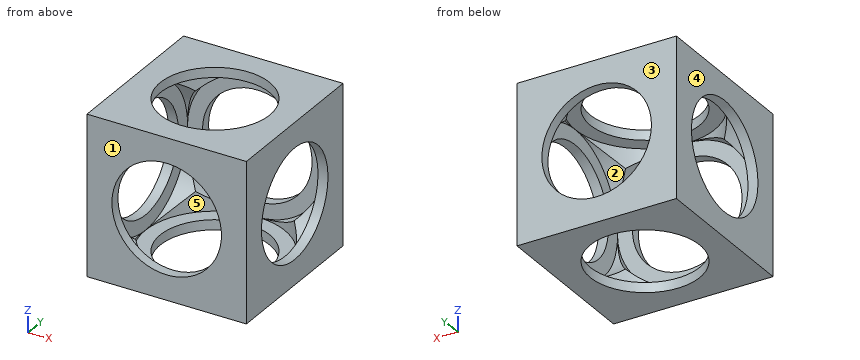
from build123d import *

# Parameters (mm, degrees)
F0_W      = 32
F0_H      = 32
F1_DEPTH  = 16
F2_R      = 11
F3_DEPTH  = 32.001
F4_R      = 11
F5_DEPTH  = 32.001
F6_R      = 11
F7_DEPTH  = 32.001
F8_R      = 14
F9_DEPTH  = 14
F10_R     = 14
F11_DEPTH = 14
F12_R     = 14
F13_DEPTH = 14


with BuildPart() as f1:
    # F0 (on Top) → F1 (new body, symmetric)
    with BuildSketch(Plane.XY):
        Rectangle(F0_W, F0_H)
    extrude(amount=F1_DEPTH, both=True)

    # F2 (on face) → F3 (cut, through all)
    with BuildSketch(Plane(origin=(-16, 0, 0), x_dir=(0, -1, 0), z_dir=(-1, 0, 0))):
        Circle(F2_R)
    extrude(amount=-F3_DEPTH, mode=Mode.SUBTRACT)

    # F4 (on face) → F5 (cut, through all)
    with BuildSketch(Plane.XY.offset(16)):
        Circle(F4_R)
    extrude(amount=-F5_DEPTH, mode=Mode.SUBTRACT)

    # F6 (on face) → F7 (cut, through all)
    with BuildSketch(Plane(origin=(0, 16, 0), x_dir=(-1, 0, 0), z_dir=(0, 1, 0))):
        Circle(F6_R)
    extrude(amount=-F7_DEPTH, mode=Mode.SUBTRACT)

    # F8 (on Top) → F9 (cut, symmetric)
    with BuildSketch(Plane.XY):
        Circle(F8_R)
    extrude(amount=F9_DEPTH, both=True, mode=Mode.SUBTRACT)

    # F10 (on Front) → F11 (cut, symmetric)
    with BuildSketch(Plane.XZ):
        Circle(F10_R)
    extrude(amount=F11_DEPTH, both=True, mode=Mode.SUBTRACT)

    # F12 (on Right) → F13 (cut, symmetric)
    with BuildSketch(Plane.YZ):
        Circle(F12_R)
    extrude(amount=F13_DEPTH, both=True, mode=Mode.SUBTRACT)


solid = f1.part
CAD build for the part. Positions are in the model's coordinates, mm. Face numbers are marked on the shaded views. A direction names the side the tool comes from. Coordinates: 2 decimals unless noted, no trailing zeros. Order: outer loops, then holes, each group sorted by start corner. A loop starts at its lowest first (then second) coordinate and runs counter-clockwise, first axis right, second up. Notation, with made-up numbers: (72.5, 68) -> (120.5, 68) arc R29 ccw to (120.5, 103) -> close; hole circle Ø11 at (9, 80.25). An arc over 180 degrees is marked (long way). Answer in a Markdown table with one row per item.
1) Band-saw the part on C-C (y = -12.5). List the corners of the cut face in (x, z).
Check values:
| item | result |
|---|---|
| outline | (-16, -16) -> (16, -16) -> (16, 16) -> (-16, 16) -> close; hole (-14, -6.3) -> (-12.5, -6.3) arc R14 ccw to (-6.3, -12.5) -> (-6.3, -14) -> (6.3, -14) -> (6.3, -12.5) arc R14 ccw to (12.5, -6.3) -> (14, -6.3) -> (14, 6.3) -> (12.5, 6.3) arc R14 ccw to (6.3, 12.5) -> (6.3, 14) -> (-6.3, 14) -> (-6.3, 12.5) arc R14 ccw to (-12.5, 6.3) -> (-14, 6.3) -> close |
2) Mould opens along Y. For the marked faces 1, 2 and 3 say: pulls with the +Y half, pulls with the -Y half, needs draft (parallel to the pull), parting line crosses it, or undercut.
Check values:
| item | result |
|---|---|
| face 1 | pulls with the -Y half |
| face 2 | undercut |
| face 3 | pulls with the +Y half |
3) Drill centre lines: line 1 (Y direction, x = -11, z = 2); line 2 (Y direction, x = -14.7, z = 0). Where is each one in solid material? Low to high.
Check values:
| item | result |
|---|---|
| line 1 | -16 to -14, 14 to 16 |
| line 2 | -16 to -11, 11 to 16 |
4) Band-saw the part on A-A (z = 2). Give the number of separate pieces and of enclosed holes in the cut face, and give its area (3 significant figures).
Check values:
| item | result |
|---|---|
| separate pieces | 4 |
| enclosed holes | 0 |
| area | 67.0 mm2 |
5) Flat gauge pins, fed straight in: P1, Ø8, axis at y = 7, z = -3.5, coming from the +X side; P2, Ø1, axis at x = 7, z = -5, coming from the +Y side. Where does each tip first touch, or does it go through?
Check values:
| item | result |
|---|---|
| P1 | x = 16 |
| P2 | through |
6) Band-saw the part on D-D (z = -13). List the corners of the cut face in (x, y), and give its area (3 significant figures).
Check values:
| item | result |
|---|---|
| outline | (-16, -16) -> (16, -16) -> (16, 16) -> (-16, 16) -> close; hole (-14, -5.2) -> (-13, -5.2) arc R14 ccw to (-5.2, -13) -> (-5.2, -14) -> (5.2, -14) -> (5.2, -13) arc R14 ccw to (13, -5.2) -> (14, -5.2) -> (14, 5.2) -> (13, 5.2) arc R14 ccw to (5.2, 13) -> (5.2, 14) -> (-5.2, 14) -> (-5.2, 13) arc R14 ccw to (-13, 5.2) -> (-14, 5.2) -> close |
| area | 395 mm2 |
7) Which spindle directions (+Z, -Z, +X, -X, +Y, -Y) get a long thin tool onto all of the face, cutting with end or side? Do the marked faces 4 and 5. Say none if no direction does.
Check values:
| item | result |
|---|---|
| face 4 | +Z, -Z, -X, +Y, -Y |
| face 5 | none |
